Input: part model. Units: mm. Frame: model coordinates. Face numbers are marked on the shaded views. A direction names the side the tool comes from. Round coordinates to 2 decimals unless told otherwise and drop trailing zeros. Write each loop counter-clockwise with the first axis right and the second up, starting at its lowest first coordinate (ties: lowest second). Pieces come first, ordered by that corner, then holes. Notation, with made-up numbers: (4, -22) - (47, -22) arc R14 cw to (47, 2) - close; hole circle Ø6 at (2, 20). An arc over 180 degrees is marked (long way). One line per item, written item: value. Start each with the question number.
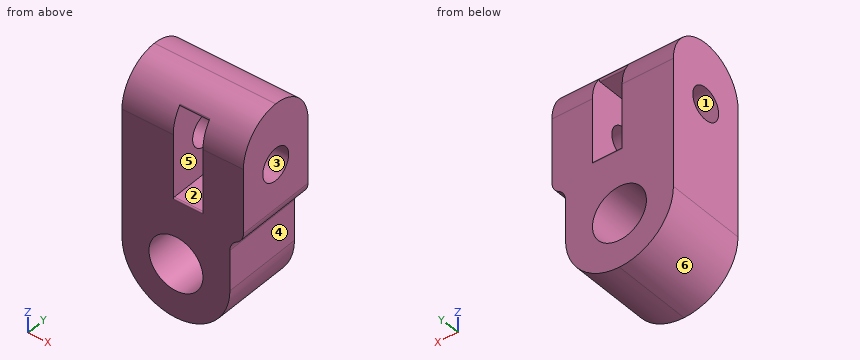
```python
from build123d import *

# Parameters (mm, degrees)
SKETCH1_R           = 2.54
BOSS_EXTRUDE1_DEPTH = 7.62
SKETCH2_R           = 1.524
CUT_EXTRUDE1_DEPTH  = 21.993449574
FILLET1_R           = 5.08
FILLET4_R           = 3.81
FILLET2_R           = 1.27
FILLET3_R           = 1.27
SKETCH3_W           = 2.794
SKETCH3_H           = 8.128
CUT_EXTRUDE2_DEPTH  = 19.719041935
FILLET5_R           = 0.127


with BuildPart() as part:
    # Sketch1 → Boss-Extrude1 (new body)
    with BuildSketch(Plane(origin=(0, 0, 0), x_dir=(1, 0, 0), z_dir=(0, 1, 0))):
        Polygon((-5.08, 5.08), (5.08, 5.08), (5.08, -5.08), (6.35, -5.08), (6.35, -15.875), (-5.08, -15.875), align=None)
        with Locations(Location((0, 0, 0), (0, 0, 270))):
            Circle(SKETCH1_R, mode=Mode.SUBTRACT)
    extrude(amount=BOSS_EXTRUDE1_DEPTH)

    # Sketch2 → Cut-Extrude1 (cut, through all)
    with BuildSketch(Plane(origin=(6.35, 0, 0), x_dir=(0, 0, -1), z_dir=(1, 0, 0))):
        with Locations((-10.16, 3.81)):
            Circle(SKETCH2_R)
    extrude(amount=-CUT_EXTRUDE1_DEPTH, mode=Mode.SUBTRACT)

    # Fillet1
    fillet1_edges = [part.edges().sort_by_distance(p)[0] for p in [
        (-5.08, 3.81, -5.08),
        (5.08, 3.81, -5.08),
    ]]
    fillet(fillet1_edges, radius=FILLET1_R - 0.0001)  # a hair under: the kernel refuses the full size

    # Fillet4
    fillet4_edges = [part.edges().sort_by_distance(p)[0] for p in [
        (0.635, 0, 15.875),
        (0.635, 7.62, 15.875),
    ]]
    fillet(fillet4_edges, radius=FILLET4_R - 0.0001)  # a hair under: the kernel refuses the full size

    # Fillet2
    fillet2_edges = [part.edges().sort_by_distance(p)[0] for p in [
        (5.08, 3.81, 5.08),
    ]]
    fillet(fillet2_edges, radius=FILLET2_R - 0.0001)  # a hair under: the kernel refuses the full size

    # Fillet3
    fillet3_edges = [part.edges().sort_by_distance(p)[0] for p in [
        (6.35, 3.81, 5.08),
    ]]
    fillet(fillet3_edges, radius=FILLET3_R)

    # Sketch3 → Cut-Extrude2 (cut, through all)
    with BuildSketch(Plane(origin=(0, 7.62, 0), x_dir=(1, 0, 0), z_dir=(0, 1, 0))):
        with Locations((1.143, -10.16)):
            Rectangle(SKETCH3_W, SKETCH3_H)
    extrude(amount=-CUT_EXTRUDE2_DEPTH, mode=Mode.SUBTRACT)

    # Fillet5
    fillet5_edges = [part.edges().sort_by_distance(p)[0] for p in [
        (1.143, 0.670713991, 14.224),
        (1.143, 7.62, 6.096),
        (1.143, 6.949286009, 14.224),
        (1.143, 0, 6.096),
    ]]
    fillet(fillet5_edges, radius=FILLET5_R)


solid = part.part
```
Q1. Cut plane A-A, the plane z = 10.16. Output: boundary loops of the cut face in (x, y).
Q2. Contact query for flat-ended pins moving along their axis: pin 1 Ø1.1 at (y, z) = (4, 2.5) entering from +X; pin 2 Ø3 at (x, z) = (4.5, 1) entering from -Y. Output: stop coordinate, or through.
Q3. Cut plane D-D, the plane y = 2.5. Count the separate pieces of the cut face and the enclosed holes in it, and give its area (3 significant figures).
Q4. Access query for the marked faces 1 and 2. Directions: +Z, -Z, +X, -X, +Y, -Y. A direction counts if a zero-diameter tool reaches every point of the face in a straight line with its end or side. Return the directions, or none.
Q5. Material intervals for probe 1 along X at (y, z) = (6.25, 0); probe 2 along X at (y, z) = (4.5, 12.5); probe 3 along Y at (x, z) = (5.2, 10.16), sorted ascending. Write a range as from..to.
Q6. Cut plane C-C, the plane z = 13. Output: boundary loops of the cut face in (x, y).
Q7. Pull-direction query (X, two-part tool) for the marked faces 3, 4, 5 and 6; classes: pulls with the +X half, pulls with the -X half, needs draft (parallel to the pull), parting line crosses it, or undercut.
A:
1. outline: (-5.08, 0) - (-0.25, 0) - (-0.25, 2.29) - (-5.08, 2.29) - close; (-5.08, 5.33) - (-0.25, 5.33) - (-0.25, 7.62) - (-5.08, 7.62) - close; (2.54, 0) - (6.35, 0) - (6.35, 2.29) - (2.54, 2.29) - close; (2.54, 5.33) - (6.35, 5.33) - (6.35, 7.62) - (2.54, 7.62) - close
2. pin 1: stops at x = 5.08
2. pin 2: stops at y = 0
3. separate pieces: 2
3. enclosed holes: 1
3. area: 157 mm²
4. face 1: +X, -X
4. face 2: +Y, -Y
5. probe 1: x = -5.08..-2.54, 2.54..5.08
5. probe 2: x = -5.08..-0.25, 2.54..6.35
5. probe 3: y = 0..2.29, 5.33..7.62
6. outline: (-5.08, 0.12) - (-0.25, 0.12) - (-0.25, 7.5) - (-5.08, 7.5) - close; (2.54, 0.12) - (6.35, 0.12) - (6.35, 7.5) - (2.54, 7.5) - close
7. face 3: needs draft
7. face 4: pulls with the +X half
7. face 5: undercut
7. face 6: pulls with the -X half
